from build123d import *

# Parameters (mm, degrees)
F0_R     = 5
F1_DEPTH = 2
F2_DEPTH = 1
F3_DEPTH = 22
F4_SIZE2 = 0.352644
F4_SIZE  = 1.99999


# Not quite as in the source:
# - a fillet or chamfer is up to 0.001 mm smaller than in the source, because OpenCascade refuses the exact size


with BuildPart() as f1:
    # F0 (on Front) → F1 (new body)
    with BuildSketch(Plane.XZ):
        Polygon((-202.1265400052, 210), (-217.8300492651, 157.6549691337), (-92.7831770837, -310), (-52.4130318677, -310), (-194.6536201768, 221.9566717254), align=None)
        with Locations((-77.1265400052, -295)):
            Circle(F0_R, mode=Mode.SUBTRACT)
        Polygon((-182.1265400052, 242), (-194.6536201768, 221.9566717254), (-52.4130318677, -310), (227.8734599948, -310), (508.1599518573, -310), (650.4005401664, 221.9566717254), (637.8734599948, 242), (577.8734599948, 300), (477.8734599948, 350), (377.8734599948, 370), (227.8734599948, 380), (77.8734599948, 370), (-22.1265400052, 350), (-122.1265400052, 300), align=None)
        Polygon((650.4005401664, 221.9566717254), (508.1599518573, -310), (548.5300970733, -310), (673.5769692547, 157.6549691337), (657.8734599948, 210), align=None)
        with Locations((532.8734599948, -295)):
            Circle(F0_R, mode=Mode.SUBTRACT)
        Polygon((-220.1265400052, 150), (-218.1265400052, 0), (-209.1265400052, -100), (-185.1265400052, -200), (-160.1265400052, -250), (-127.1265400052, -285), (-98.1265400052, -310), (-93.8183090123, -310), (-218.3773603998, 155.8305986848), align=None)
        Polygon((674.1242803894, 155.8305986848), (549.5652290019, -310), (553.8734599948, -310), (582.8734599948, -285), (615.8734599948, -250), (640.8734599948, -200), (664.8734599948, -100), (673.8734599948, 0), (675.8734599948, 150), align=None)
        Polygon((673.5769692547, 157.6549691337), (548.5300970733, -310), (549.5652290019, -310), (674.1242803894, 155.8305986848), align=None)
        Polygon((-217.8300492651, 157.6549691337), (-218.3773603998, 155.8305986848), (-93.8183090123, -310), (-92.7831770837, -310), align=None)
    extrude(amount=F1_DEPTH)

    # F0 (on Front) → F2 (join)
    with BuildSketch(Plane.XZ):
        Polygon((-202.1265400052, 210), (-217.8300492651, 157.6549691337), (-92.7831770837, -310), (-52.4130318677, -310), (-194.6536201768, 221.9566717254), align=None)
        with Locations((-77.1265400052, -295)):
            Circle(F0_R, mode=Mode.SUBTRACT)
        Polygon((650.4005401664, 221.9566717254), (508.1599518573, -310), (548.5300970733, -310), (673.5769692547, 157.6549691337), (657.8734599948, 210), align=None)
        with Locations((532.8734599948, -295)):
            Circle(F0_R, mode=Mode.SUBTRACT)
    extrude(amount=-F2_DEPTH)

    # F0 (on Front) → F3 (join)
    with BuildSketch(Plane.XZ):
        Polygon((673.5769692547, 157.6549691337), (548.5300970733, -310), (549.5652290019, -310), (674.1242803894, 155.8305986848), align=None)
        Polygon((-217.8300492651, 157.6549691337), (-218.3773603998, 155.8305986848), (-93.8183090123, -310), (-92.7831770837, -310), align=None)
    extrude(amount=-F3_DEPTH)

    # F4 (size 2 and 0.3526539614 in the source; OpenCascade refuses exactly that, so slightly less here)
    f4_edges = [f1.edges().sort_by_distance(p)[0] for p in [
        (227.87346, -2, -310),
    ]]
    f4_side = f1.faces().sort_by_distance((227.87346, -0.533198, -310))[0]
    chamfer(f4_edges, length=F4_SIZE, length2=F4_SIZE2, reference=f4_side)


solid = f1.part
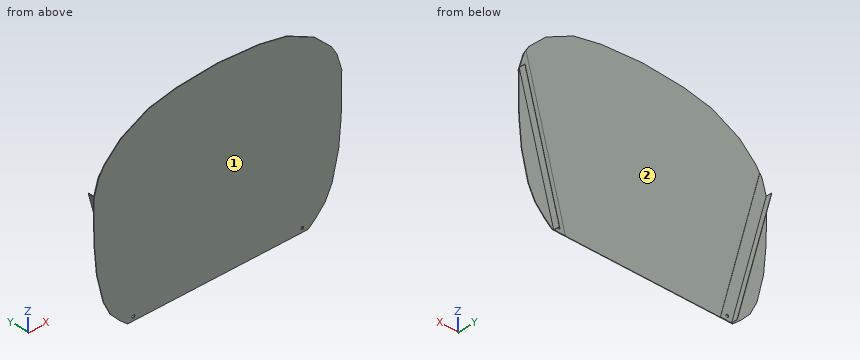
Here's how the part is built. I have some questions about the finished solid (model axes, mm). Face numbers are marked on the shaded views. A direction names the side the tool comes from. Coordinates: 2 decimals unless noted, no trailing zeros. Loops run counter-clockwise (first coordinate to the right, second up) from the corner with the lowest first, then second, coordinate; pieces in that order, holes last.
1. Imagine slicing it at B-B, the plane z = 63.5. Please give me the cut outline in (x, y), and give its area (3 significant figures).
2. I need wall thicknesses on L1, parallel to X at y = -1.1, z = -295; L2, parallel to Y at x = -121.5, z = 9; L3, parallel to X at y = 20, z = -23. Which ranges of each line are inside material? Lowest first, please.
3. For P1, Ø3, axis at y = 3.5, z = -17.5, coming from the +X side; P2, Ø1.5, axis at x = 69.5, z = 211.5, coming from the +Y side; P3, Ø16, axis at x = -77.13, z = -295, coming from the +Y side; P4, Ø16, axis at x = 532.87, z = -295, coming from the -Y side, each with a flat end and sliding along its axis, tell me the tip position at first contact or that it passes through.
4. For the marked faces 1 and 2, which set-ups out of +Z, -Z, +X, -X, +Y, -Y let a thin tool reach every point of the face, with its end or its side?
5. Imagine slicing it at A-A, the plane y = 5.5. Please give me the cut outline in (x, z).
Taken from the geometry:
1. outline: (-218.97, -2) - (674.72, -2) - (674.72, 0) - (649.44, 0) - (649.44, 22) - (648.4, 22) - (648.4, 1) - (608.03, 1) - (608.03, 0) - (-152.28, 0) - (-152.28, 1) - (-192.65, 1) - (-192.65, 22) - (-193.69, 22) - (-193.69, 0) - (-218.97, 0) - close
1. area: 1,910 mm2
2. L1: x = -115.53 to -82.13, -72.13 to 527.87, 537.87 to 571.27
2. L2: y = -2 to 0
2. L3: x = -170.56 to -169.52, 625.27 to 626.31
3. P1: stops at x = 628.18
3. P2: stops at y = 0
3. P3: stops at y = 1
3. P4: stops at y = -2
4. face 1: +Z, -Z, +X, -X, -Y
4. face 2: +Z, +Y
5. outline: (-218.38, 155.83) - (-93.82, -310) - (-92.78, -310) - (-217.83, 157.65) - close; (548.53, -310) - (549.57, -310) - (674.12, 155.83) - (673.58, 157.65) - close
